Read the model definition and answer for the solid it produces. Units are mm, in the model's axes. A direction names the side the tool comes from. Round coordinates to 2 decimals unless told otherwise and drop trailing zeros. Loops run counter-clockwise (first coordinate to the right, second up) from the corner with the lowest first, then second, coordinate; pieces in that order, holes last. Notation, with made-up numbers: M 63.5,-31.75 L 111.5,-31.75 A23 cw 111.5,-5.75 Z; hole C -19,42 d3. An arc over 180 degrees is marked long. Write each question's results on one line, items separated by ' | '.
Autodesk Inventor part; units mm, degrees
ref_plane "to_block_XY" through (0, 0, 47.5) normal (0, 0, 1) x (1, 0, 0)
ref_plane "to_block_YZ" through (0, 0, 47.5) normal (1, 0, 0) x (0, 1, 0)
ref_plane "to_block_ZX" through (0, 0, 47.5) normal (0, 1, 0) x (0, 0, 1)
sketch "_____2" plane through (0, 0, 0) normal (0, 0, 1) x (1, 0, 0)
  line L0 (-10, 1.8) -> (-10, 0)
  line L1 (-10, 0) -> (10, 0)
  line L2 (10, 0) -> (10, 1.8)
  line L3 (10, 1.8) -> (8.9929, 2.8071)
  line L4 (8.9929, 2.8071) -> (7.508, 1.3222)
  line L5 (7.508, 1.3222) -> (4.6795, 4.1506)
  line L6 (4.6795, 4.1506) -> (5.8109, 5.282)
  arc A0 (5.8109, 5.282) -> (5.8109, 5.5648) centre (5.6695, 5.4234) ccw
  line L7 (5.8109, 5.5648) -> (3.9343, 7.4414)
  arc A1 (3.9343, 7.4414) -> (3.7929, 7.5) centre (3.7929, 7.3) ccw
  line L8 (3.7929, 7.5) -> (-3.7929, 7.5)
  arc A2 (-3.7929, 7.5) -> (-3.9343, 7.4414) centre (-3.7929, 7.3) ccw
  line L9 (-3.9343, 7.4414) -> (-5.8109, 5.5648)
  arc A3 (-5.8109, 5.5648) -> (-5.8109, 5.282) centre (-5.6695, 5.4234) ccw
  line L10 (-5.8109, 5.282) -> (-4.6795, 4.1506)
  line L11 (-4.6795, 4.1506) -> (-7.508, 1.3222)
  line L12 (-7.508, 1.3222) -> (-8.9929, 2.8071)
  line L13 (-8.9929, 2.8071) -> (-10, 1.8)
extrude "Extrusion1" add sketch "_____2" along normal blind 95
sketch "Sketch2" plane through (-3.7929, 7.5, 0) normal (0, 1, 0) x (1, 0, 0)
  point P0 (3.7929, -7.5)
hole "Hole1" at (0, 7.5, 7.5) direction (0, -1, 0) diameter 3.5 depth 7.5 counterbore diameter 6 counterbore depth 4
pattern_linear "Rectangular Pattern1" count 3 spacing 40 along (0, 0, 1) of "Hole1"
ref_plane "to_block_XY" through (0, 0, 47.5) normal (0, 0, 1) x (1, 0, 0)
ref_plane "to_block_YZ" through (0, 0, 47.5) normal (1, 0, 0) x (0, 1, 0)
ref_plane "to_block_ZX" through (0, 0, 47.5) normal (0, 1, 0) x (0, 0, 1)
ref_plane "to_block2_XY" through (0, 0, 47.5) normal (0, 0, 1) x (1, 0, 0)
ref_plane "to_block2_YZ" through (0, 0, 47.5) normal (1, 0, 0) x (0, 1, 0)
ref_plane "to_block2_ZX" through (0, 0, 47.5) normal (0, 1, 0) x (0, 0, 1)
properties part number "JKSGR10-95"
1. Find section B-B, the plane z = 7.5. Give the vertices of the cut face in (x, y), then the cut area to 3 significant figures.
Completed:
outline: M -10,0 L -1.75,0 L -1.75,3.5 L -3,3.5 L -3,7.5 L -3.79,7.5 A0.2 ccw -3.93,7.44 L -5.81,5.56 A0.2 ccw -5.81,5.28 L -4.68,4.15 L -7.51,1.32 L -8.99,2.81 L -10,1.8 Z; M 1.75,0 L 10,0 L 10,1.8 L 8.99,2.81 L 7.51,1.32 L 4.68,4.15 L 5.81,5.28 A0.2 ccw 5.81,5.56 L 3.93,7.44 A0.2 ccw 3.79,7.5 L 3,7.5 L 3,3.5 L 1.75,3.5 Z | area: 62.8 mm2
2. Find section C-C, the plane z = 64. Give the vertices of the cut face in (x, y), then the cut area to 3 significant figures.
Completed:
outline: M -10,0 L 10,0 L 10,1.8 L 8.99,2.81 L 7.51,1.32 L 4.68,4.15 L 5.81,5.28 A0.2 ccw 5.81,5.56 L 3.93,7.44 A0.2 ccw 3.79,7.5 L -3.79,7.5 A0.2 ccw -3.93,7.44 L -5.81,5.56 A0.2 ccw -5.81,5.28 L -4.68,4.15 L -7.51,1.32 L -8.99,2.81 L -10,1.8 Z | area: 99.0 mm2
3. Determine the mould class of faces 1 (the face through (2, 3.5, 87)), 2 (the face through (-0.1, 5.5, 84.5)), 3 (the face through (0, 3, 95)), 4 (the face through (-6.07, 2.76, 46.84)) for opening direction Z: released by +Z, released by -Z, zero draft, split by the parting line, or undercut.
Completed:
face 1: undercut | face 2: undercut | face 3: released by +Z | face 4: zero draft
4. Find section A-A, the plane x = 0. Give the vertices of the cut face in (y, z).
Completed:
outline: M 0,0 L 7.5,0 L 7.5,4.5 L 3.5,4.5 L 3.5,5.75 L 0,5.75 Z; M 0,9.25 L 3.5,9.25 L 3.5,10.5 L 7.5,10.5 L 7.5,44.5 L 3.5,44.5 L 3.5,45.75 L 0,45.75 Z; M 0,49.25 L 3.5,49.25 L 3.5,50.5 L 7.5,50.5 L 7.5,84.5 L 3.5,84.5 L 3.5,85.75 L 0,85.75 Z; M 0,89.25 L 3.5,89.25 L 3.5,90.5 L 7.5,90.5 L 7.5,95 L 0,95 Z
5. Given P1, Ø3, axis at x = 6.5, y = 3.5, coming from the +Z side, flat-ended and moving along its own axis, determine where the tip first touches the part or whether it passes through.
Completed:
P1: stops at z = 95
6. Which of the six approach directions +Z, -Z, +X, -X, +Y, -Y give full straight-line access (tool end or side, diameter ignored) to faces 5 (the face through (6.11, 2.72, 46.84)), 6 (the face through (2, 3.5, 7)), 7 (the face through (-8.24, 2.054, 46.835)), 8 (the face through (-4.859, 6.516, 46.835))?
Completed:
face 5: +Z, -Z | face 6: +Y | face 7: +Z, -Z, +Y | face 8: +Z, -Z, -X, +Y
7. Find the intervals of material crossed by L1, parallel to Z at x = 0, y = 1.5; L2, parallel to Z at x = -1, y = 1.25; L3, parallel to X at y = 2.3, z = 7.5, in increasing order.
Completed:
L1: z = 0 to 5.75, 9.25 to 45.75, 49.25 to 85.75, 89.25 to 95 | L2: z = 0 to 6.06, 8.94 to 46.06, 48.94 to 86.06, 88.94 to 95 | L3: x = -9.5 to -8.49, -6.53 to -1.75, 1.75 to 6.53, 8.49 to 9.5
